Here's how the part is built. I have some questions about the finished solid (model axes, mm). Face numbers are marked on the shaded views. A direction names the side the tool comes from. Give positions to 0.01 mm unless a question says otherwise; leave off trailing zeros. Loops run counter-clockwise (first coordinate to the right, second up) from the corner with the lowest first, then second, coordinate; pieces in that order, holes last. Notation, with made-up numbers: M -7.5,40 L 38.5,40 A34 cw 38.5,75 Z; hole C 32.25,9 d5. An arc over 180 degrees is marked long. Answer as CSV lines item,"result". Start each with the question number.
Item 1: If we mould it in two halves opening along X, with no side actions, what happens to the marked faces 3, 4 and 5? For each: released by +X, released by -X, zero draft, split by the parting line, or undercut.
Item 2: I want a section at B-B on x = 5. List the corners of the cut face in (y, z) for me, plus the area to 3 significant figures.
Item 3: I want a section at C-C on z = 4.25. List the corners of the cut face in (x, y) for me.
Item 4: For the marked faces 1 and 2, which set-ups out of +Z, -Z, +X, -X, +Y, -Y let a thin tool reach every point of the face, with its end or its side?
Item 5: Will these pins go through, and if not, where does the flat tip stop? P1, Ø2, axis at y = 4, z = 14, coming from the -X side; P2, Ø10, axis at x = 1.5, z = 16.5, coming from the -Y side; P3, Ø1.5, axis at x = 0, y = -0.5, coming from the -Z side; P4, Ø19, axis at x = 3.5, y = 1.5, coming from the +Z side.
Item 6: If I drill on line 1 along Y through (x, z) = (0, 4.25); line 2 along Z through (x, y) = (-13, 13.5); line 3 along Z through (x, y) = (-1, -4), over which ranges is the centre line in solid material (lowest first)? Write a range as from..to.
Item 7: I want a section at A-A on y = 0. List the corners of the cut face in (x, z) for me, plus the area to 3 significant figures.
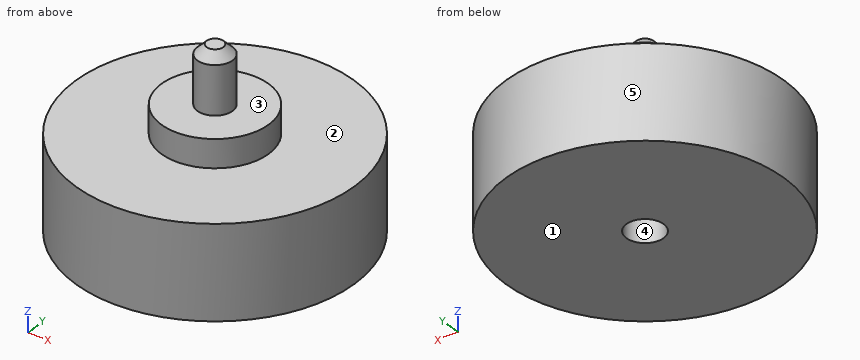
from build123d import *

# Parameters (mm, degrees)
F2_SIZE = 1.27


with BuildPart() as f1:
    # F0 (on Front) → F1 (revolve)
    with BuildSketch(Plane.XZ):
        Polygon((2.54, 0), (19.05, 0), (19.05, 12.7), (7.3406, 12.7), (7.3406, 16.51), (2.413, 16.51), (2.413, 24.3586), (0, 24.3586), (0, 16.51), (0, 12.7), (0, 7.874), (2.54, 7.874), align=None)
    revolve(axis=Axis((0, 0, 14.605), (0, 0, 1)))

    # F2
    f2_edges = [f1.edges().sort_by_distance(p)[0] for p in [
        (-2.413, 0, 24.3586),
    ]]
    chamfer(f2_edges, length=F2_SIZE)


solid = f1.part
Result:
1,face 3,"zero draft"
1,face 4,"undercut"
1,face 5,"split by the parting line"
2,outline,"M -18.38,0 L 18.38,0 L 18.38,12.7 L 5.37,12.7 L 5.37,16.51 L -5.37,16.51 L -5.37,12.7 L -18.38,12.7 Z"
2,area,"508 mm^2"
3,outline,"C 0,0 d38.1; hole C 0,0 d5.08"
4,face 1,"-Z, +X, -X, +Y, -Y"
4,face 2,"+Z"
5,P1,"x = -6.7"
5,P2,"y = -19.05"
5,P3,"z = 7.87"
5,P4,"z = 24.36"
6,line 1,"-19.05..-2.54, 2.54..19.05"
6,line 2,"0..12.7"
6,line 3,"0..16.51"
7,outline,"M -19.05,0 L -2.54,0 L -2.54,7.87 L 2.54,7.87 L 2.54,0 L 19.05,0 L 19.05,12.7 L 7.34,12.7 L 7.34,16.51 L 2.41,16.51 L 2.41,23.09 L 1.14,24.36 L -1.14,24.36 L -2.41,23.09 L -2.41,16.51 L -7.34,16.51 L -7.34,12.7 L -19.05,12.7 Z"
7,area,"536 mm^2"
